Here's how the part is built. I have some questions about the finished solid (model axes, mm). Face numbers are marked on the shaded views. A direction names the side the tool comes from. Round coordinates to 2 decimals unless told otherwise and drop trailing zeros. Answer as a JSON object with one key per item and string values.
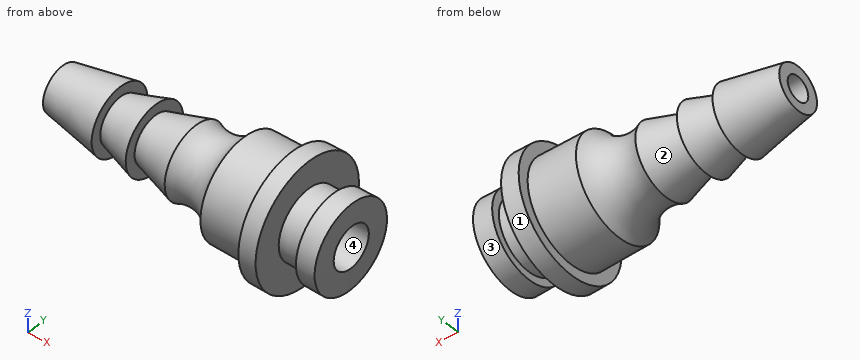
from build123d import *


with BuildPart() as part:
    # Sketch1 → Revolve1 (revolve)
    with BuildSketch(Plane(origin=(0, 0, 0), x_dir=(1, 0, 0), z_dir=(0, 1, 0))):
        with BuildLine():
            Line((-11.493478261, -0.960869565), (1.406521739, -0.960869565))
            Line((1.406521739, -0.960869565), (1.826198847, -1.279930678))
            Line((1.826198847, -1.279930678), (8.484993151, -1.279930678))
            Line((8.484993151, -1.279930678), (8.474039616, -2.818617799))
            Line((8.474039616, -2.818617799), (7.16746221, -2.818617799))
            Line((7.16746221, -2.818617799), (7.174039616, -2.247384123))
            Line((7.174039616, -2.247384123), (5.474039616, -2.247384123))
            Line((5.474039616, -2.247384123), (5.486521739, -4.139307546))
            Line((5.486521739, -4.139307546), (4.284364062, -4.139307546))
            Line((4.284364062, -4.139307546), (4.286521739, -3.385626586))
            Line((4.286521739, -3.385626586), (0.986521739, -3.385626586))
            ThreePointArc((0.986521739, -3.385626586), (-0.48998153, -2.304776001), (-2.313478261, -2.456958665))
            Line((-2.313478261, -2.456958665), (-5.093478261, -1.670869565))
            Line((-5.093478261, -1.670869565), (-5.093478261, -2.391060827))
            Line((-5.093478261, -2.391060827), (-7.493478261, -1.670869565))
            Line((-7.493478261, -1.670869565), (-7.499524272, -2.359905691))
            Line((-7.499524272, -2.359905691), (-11.493478261, -1.670869565))
            Line((-11.493478261, -1.670869565), (-11.493478261, -0.960869565))
        make_face()
    revolve(axis=Axis((-11.493478261, 0, 0.110869565), (0.9999010425950651, 0, -0.014067871811395011)))


solid = part.part
Item 1: I want a section at A-A on y = 1.75. Count the separate pieces of the cut face and the enclosed holes in it, plus the area to 3 significant figures.
Solution:
{"separate pieces": "3", "enclosed holes": "0", "area": "68.0 mm2"}
Item 2: For P1, Ø4, axis at x = 0, y = -1, coming from the -Z side; P2, Ø4, axis at x = 0.5, z = 3, coming from the -Y side; P3, Ø1.5, axis at x = -5.5, y = -1.5, coming from the +Z side, each with a flat end and sliding along its axis, tell me the tip position at first contact or that it passes through.
Solution:
{"P1": "stops at z = -3.54", "P2": "stops at y = -3.26", "P3": "stops at z = 2.23"}
Item 3: If I drill on L1, parallel to Z at x = 2, y = 0.75; L2, parallel to Z at x = 7.25, y = -1.75; L3, parallel to Y at x = -5.75, z = 0.5, over which ranges is the centre line in solid material (lowest first)? Write a range as from..to.
Solution:
{"L1": "z = -3.46..-1.21, 1.05..3.3", "L2": "z = -2.56..2.25", "L3": "y = -2.12..-0.8, 0.8..2.12"}
Item 4: We'd pull the mould along Y, two halves only. Please class the marked faces 3 and 4: +Y half, -Y half, draft (parallel to the pull), parting line (faces both ways), or undercut.
Solution:
{"face 3": "parting line", "face 4": "undercut"}
Item 5: For the marked faces 1 and 2, which set-ups out of +Z, -Z, +X, -X, +Y, -Y let a thin tool reach every point of the face, with its end or its side?
Solution:
{"face 1": "-X", "face 2": "none"}
